Source: CAD feature listing. Evaluate the final solid. Frame: model axes, mm. Give positions to 0.01 mm unless a question says otherwise; leave off trailing zeros. Write each loop counter-clockwise with the first axis right and the second up, starting at its lowest first coordinate (ties: lowest second). Pieces come first, ordered by that corner, then holes. Notation, with made-up numbers: (-15.75, -38) -> (32.25, -38) arc R6 ccw to (32.25, -29) -> close; hole circle Ø9 at (12.25, -13.75). An arc over 180 degrees is marked (long way). Answer as a JSON object with one key per item and string values. Group by question number.
Item 1: Section query C-C on z = 2.8. Return the cut outline in (x, y), plus the area to 3 significant figures.
Item 2: Section query D-D on y = -25. Return the cut outline in (x, z).
Item 3: Section query A-A on y = 0. Return the cut outline in (x, z).
Item 4: Ray query, probe 1 along Y at (x, z) = (0, 3.45); probe 2 along Y at (x, z) = (-25, 1.3); probe 3 along Y at (x, z) = (-60, 1). Return the intervals inside material, ascending. Write a range as from..to.
Item 5: Section query B-B on x = 0. Return the cut outline in (y, z), plus the area to 3 significant figures.
Item 6: First-contact query: pin 1 Ø2 at (x, y) = (25, 0) entering from +Z. Flat tip, straight axial feed; report the tip coordinate or a pass-through.
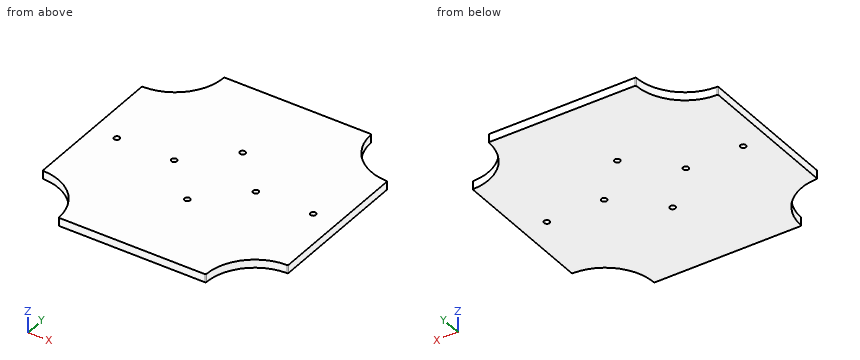
from build123d import *

# Parameters (mm, degrees)
ESQUISSE1_W             = 150
ESQUISSE1_H             = 150
BOSS_EXTRU_1_DEPTH      = 5
ENL_V_MAT_EXTRU_1_DEPTH = 5
D_GAGEMENT_M31_D        = 3.4
CONG_1_R                = 0.5


with BuildPart() as part:
    # Esquisse1 → Boss.-Extru.1 (new body)
    with BuildSketch(Plane.XY):
        Rectangle(ESQUISSE1_W, ESQUISSE1_H)
    extrude(amount=BOSS_EXTRU_1_DEPTH)

    # Esquisse2 → Enlèv. mat.-Extru.1 (cut)
    with BuildSketch(Plane.XY.offset(5)):
        with BuildLine():
            Line((45, 75), (75, 75))
            Line((75, 75), (75, 45))
            ThreePointArc((75, 45), (53.786796564, 53.786796564), (45, 75))
        make_face()
        with BuildLine():
            Line((75, -75), (45, -75))
            ThreePointArc((45, -75), (53.786796564, -53.786796564), (75, -45))
            Line((75, -45), (75, -75))
        make_face()
        with BuildLine():
            Line((-75, -75), (-75, -45))
            ThreePointArc((-75, -45), (-53.786796564, -53.786796564), (-45, -75))
            Line((-45, -75), (-75, -75))
        make_face()
        with BuildLine():
            Line((-75, 75), (-45, 75))
            ThreePointArc((-45, 75), (-53.786796564, 53.786796564), (-75, 45))
            Line((-75, 45), (-75, 75))
        make_face()
    extrude(amount=-ENL_V_MAT_EXTRU_1_DEPTH, mode=Mode.SUBTRACT)

    # Dégagement M31 (through all)
    with Locations(Plane(origin=(0, 0, 0), x_dir=(-1, 0, 0), z_dir=(0, 0, -1))):
        with Locations((0, 25), (0, -25), (60, 0), (25, 0), (-25, 0), (-60, 0)):
            Hole(D_GAGEMENT_M31_D / 2)

    # Congé1
    cong_1_edges = [part.edges().sort_by_distance(p)[0] for p in [
        (-75, 45, 2.5),
        (-45, 75, 2.5),
        (-45, -75, 2.5),
        (-75, -45, 2.5),
        (75, -45, 2.5),
        (45, -75, 2.5),
        (75, 45, 2.5),
        (45, 75, 2.5),
    ]]
    fillet(cong_1_edges, radius=CONG_1_R)


solid = part.part
Worked answers:
{
 "1": {"outline": "(-75, -44.5) arc R0.5 ccw to (-74.51, -45) arc R30 cw to (-45, -74.51) arc R0.5 ccw to (-44.5, -75) -> (44.5, -75) arc R0.5 ccw to (45, -74.51) arc R30 cw to (74.51, -45) arc R0.5 ccw to (75, -44.5) -> (75, 44.5) arc R0.5 ccw to (74.51, 45) arc R30 cw to (45, 74.51) arc R0.5 ccw to (44.5, 75) -> (-44.5, 75) arc R0.5 ccw to (-45, 74.51) arc R30 cw to (-74.51, 45) arc R0.5 ccw to (-75, 44.5) -> close; hole circle Ø3.4 at (-60, 0); hole circle Ø3.4 at (-25, 0); hole circle Ø3.4 at (0, -25); hole circle Ø3.4 at (0, 25); hole circle Ø3.4 at (25, 0); hole circle Ø3.4 at (60, 0)", "area": "19,600 mm^2"},
 "2": {"outline": "(-75, 0) -> (-1.7, 0) -> (-1.7, 5) -> (-75, 5) -> close; (1.7, 0) -> (75, 0) -> (75, 5) -> (1.7, 5) -> close"},
 "3": {"outline": "(-75, 0) -> (-61.7, 0) -> (-61.7, 5) -> (-75, 5) -> close; (-58.3, 0) -> (-26.7, 0) -> (-26.7, 5) -> (-58.3, 5) -> close; (-23.3, 0) -> (23.3, 0) -> (23.3, 5) -> (-23.3, 5) -> close; (26.7, 0) -> (58.3, 0) -> (58.3, 5) -> (26.7, 5) -> close; (61.7, 0) -> (75, 0) -> (75, 5) -> (61.7, 5) -> close"},
 "4": {"probe 1": "-75..-26.7, -23.3..23.3, 26.7..75", "probe 2": "-75..-1.7, 1.7..75", "probe 3": "-49.02..-1.7, 1.7..49.02"},
 "5": {"outline": "(-75, 0) -> (-26.7, 0) -> (-26.7, 5) -> (-75, 5) -> close; (-23.3, 0) -> (23.3, 0) -> (23.3, 5) -> (-23.3, 5) -> close; (26.7, 0) -> (75, 0) -> (75, 5) -> (26.7, 5) -> close", "area": "716 mm^2"},
 "6": {"pin 1": "through"}
}
